from build123d import *

# Parameters (mm, degrees)
S_BOX1_W     = 22.8
S_BOX1_H     = 12.2
BOSS_1_DEPTH = 28.4
S_BOX2_W     = 32.8
S_BOX2_H     = 12.2
BOSS_2_DEPTH = 2.5
S_CYL3_R     = 2.4
BOSS_3_DEPTH = 4.5


with BuildPart() as part:
    # S_box1 → Boss_1 (new body)
    with BuildSketch(Plane.XY.offset(-32.4)):
        with Locations((5.6, 0)):
            Rectangle(S_BOX1_W, S_BOX1_H)
    extrude(amount=BOSS_1_DEPTH)

    # S_box2 → Boss_2 (add)
    with BuildSketch(Plane.XY.offset(-14)):
        with Locations((5.6, 0)):
            Rectangle(S_BOX2_W, S_BOX2_H)
    extrude(amount=BOSS_2_DEPTH)

    # S_cyl3 → Boss_3 (add)
    with BuildSketch(Plane.XY.offset(-4.5)):
        Circle(S_CYL3_R)
    extrude(amount=BOSS_3_DEPTH)


solid = part.part
Can you work these out from the model? Positions are in its coordinate system, mm. A direction names the side the tool comes from. Round coordinates to 2 decimals unless told otherwise and drop trailing zeros. Order: outer loops, then holes, each group sorted by start corner. A loop starts at its lowest first (then second) coordinate and runs counter-clockwise, first axis right, second up. Notation, with made-up numbers: M -4,46.5 L 1,46.5 A22 ccw 1,61.5 Z; hole C 59.5,-0.75 d7. An arc over 180 degrees is marked long. Use a Markdown table: item, result.
1) Imagine slicing it at D-D (y = 0). List the corners of the cut face in (x, z) for me, then the cut area to 3 significant figures.
Geometry says:
| item | result |
|---|---|
| outline | M -10.8,-14 L -5.8,-14 L -5.8,-32.4 L 17,-32.4 L 17,-14 L 22,-14 L 22,-11.5 L 17,-11.5 L 17,-4 L 2.4,-4 L 2.4,0 L -2.4,0 L -2.4,-4 L -5.8,-4 L -5.8,-11.5 L -10.8,-11.5 Z |
| area | 692 mm² |
2) Imagine slicing it at B-B (y = 3). List the corners of the cut face in (x, z) for me.
Geometry says:
| item | result |
|---|---|
| outline | M -10.8,-14 L -5.8,-14 L -5.8,-32.4 L 17,-32.4 L 17,-14 L 22,-14 L 22,-11.5 L 17,-11.5 L 17,-4 L -5.8,-4 L -5.8,-11.5 L -10.8,-11.5 Z |
3) Imagine slicing it at C-C (z = -20). List the corners of the cut face in (x, y) for me, then the cut area to 3 significant figures.
Geometry says:
| item | result |
|---|---|
| outline | M -5.8,-6.1 L 17,-6.1 L 17,6.1 L -5.8,6.1 Z |
| area | 278 mm² |
4) Imagine slicing it at A-A (x = 0). List the corners of the cut face in (y, z) for me.
Geometry says:
| item | result |
|---|---|
| outline | M -6.1,-32.4 L 6.1,-32.4 L 6.1,-4 L 2.4,-4 L 2.4,0 L -2.4,0 L -2.4,-4 L -6.1,-4 Z |
5) I'm going to push flat-ended pins straight in: P1, Ø4, axis at y = 1, z = -9, coming from the +X side; P2, Ø3.5, axis at y = -1.5, z = -19, coming from the -X side; P3, Ø4, axis at x = 19.5, y = 2.5, coming from the +Z side. Where does each tip first touch, or does it pass through?
Geometry says:
| item | result |
|---|---|
| P1 | stops at x = 17 |
| P2 | stops at x = -5.8 |
| P3 | stops at z = -11.5 |
6) On a 3-axis mill with a long thin cutter (end or side, diameter ignored), from which of +Z, -Z, +X, -X, +Y, -Y can I reach the whole of each face in a straight line? I mean faces 1 (the face through (-8, 0, -11.5)), 2 (the face through (17, 0, -23)), 3 (the face through (1.29, 2.024, -2.028)). Say none if no direction works.
Geometry says:
| item | result |
|---|---|
| face 1 | +Z, -X, +Y, -Y |
| face 2 | -Z, +X, +Y, -Y |
| face 3 | +Z |
7) If I drill on line 1 along Z through (x, y) = (-9, 0.75); line 2 along X through (y, z) = (-3.75, -26); line 3 along Z through (x, y) = (7.5, 2.5), over which ranges is the centre line in solid material (lowest first)?
Geometry says:
| item | result |
|---|---|
| line 1 | z = -14 to -11.5 |
| line 2 | x = -5.8 to 17 |
| line 3 | z = -32.4 to -4 |
